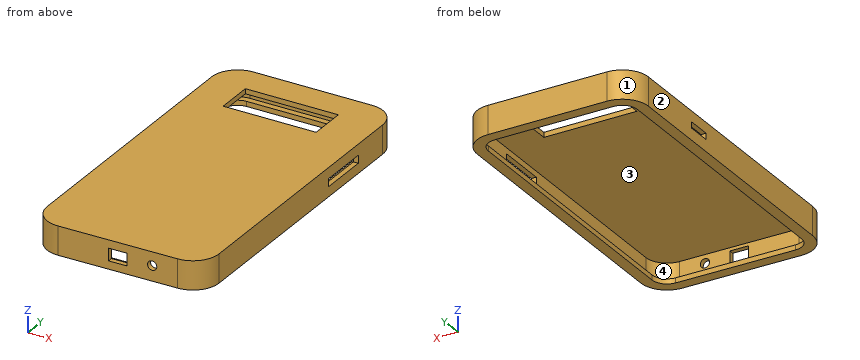
from build123d import *

# Parameters (mm, degrees)
F0_W       = 38.1
F0_H       = 15.24
F1_DEPTH   = 7.62
F2_W       = 20.32
F2_H       = 3.1982096843
F3_DEPTH   = 25.4
F5_W       = 10.16
F5_H       = 2.54
F6_DEPTH   = 25.4
F4_W       = 3.81
F4_H       = 5.08
F4_R       = 1.8758350377
F7_DEPTH   = 25.4
F8_DEPTH   = 7.62
F1_FACE3_W = 38.1
F1_FACE3_H = 15.24
F9_DEPTH   = 2.032
F10_DEPTH  = 2.032


with BuildPart() as f1:
    # F0 (on Top) → F1 (new body)
    with BuildSketch(Plane.XY):
        with BuildLine():
            Line((15.0151342493, 51.7147295177), (-33.7528657507, 51.7147295177))
            ThreePointArc((-33.7528657507, 51.7147295177), (-39.8594399131, 49.18530368), (-42.3888657507, 43.0787295177))
            Line((-42.3888657507, 43.0787295177), (-42.3888657507, -69.7396477934))
            ThreePointArc((-42.3888657507, -69.7396477934), (-39.8300752503, -75.8754460869), (-33.6700096372, -78.3752503123))
            Line((-33.6700096372, -78.3752503123), (15.0979903628, -77.9073354291))
            ThreePointArc((15.0979903628, -77.9073354291), (21.1509325427, -75.3489424097), (23.6511342493, -69.2717329101))
            Line((23.6511342493, -69.2717329101), (23.6511342493, 43.0787295177))
            ThreePointArc((23.6511342493, 43.0787295177), (21.1217084116, 49.18530368), (15.0151342493, 51.7147295177))
        make_face()
        with BuildLine():
            ThreePointArc((-39.8488657507, 43.0787295177), (-38.0633886888, 47.3892524558), (-33.7528657507, 49.1747295177))
            Line((-33.7528657507, 49.1747295177), (15.0151342493, 49.1747295177))
            ThreePointArc((15.0151342493, 49.1747295177), (19.3256571874, 47.3892524558), (21.1111342493, 43.0787295177))
            Line((21.1111342493, 43.0787295177), (21.1111342493, -69.2717329101))
            ThreePointArc((21.1111342493, -69.2717329101), (19.3462859858, -73.561527851), (15.0736209176, -75.3674523353))
            Line((15.0736209176, -75.3674523353), (-33.6943790824, -75.8353672185))
            ThreePointArc((-33.6943790824, -75.8353672185), (-38.0426606916, -74.07079953), (-39.8488657507, -69.7396477934))
            Line((-39.8488657507, -69.7396477934), (-39.8488657507, 43.0787295177))
        make_face(mode=Mode.SUBTRACT)
        with BuildLine():
            Line((15.0151342493, 49.1747295177), (-33.7528657507, 49.1747295177))
            ThreePointArc((-33.7528657507, 49.1747295177), (-38.0633886888, 47.3892524558), (-39.8488657507, 43.0787295177))
            Line((-39.8488657507, 43.0787295177), (-39.8488657507, -69.7396477934))
            ThreePointArc((-39.8488657507, -69.7396477934), (-38.0426606916, -74.07079953), (-33.6943790824, -75.8353672185))
            Line((-33.6943790824, -75.8353672185), (15.0736209176, -75.3674523353))
            ThreePointArc((15.0736209176, -75.3674523353), (19.3462859858, -73.561527851), (21.1111342493, -69.2717329101))
            Line((21.1111342493, -69.2717329101), (21.1111342493, 43.0787295177))
            ThreePointArc((21.1111342493, 43.0787295177), (19.3256571874, 47.3892524558), (15.0151342493, 49.1747295177))
        make_face()
        with Locations((-10.6388657507, 33.9347295177)):
            Rectangle(F0_W, F0_H, mode=Mode.SUBTRACT)
    extrude(amount=F1_DEPTH)

    # F2 (on face) → F3 (join)
    with BuildSketch(Plane.YZ.offset(23.6511342493)):
        with Locations((16.1547295177, 3.6192152184)):
            Rectangle(F2_W, F2_H)
    extrude(amount=F3_DEPTH)

    # F5 (on face) → F6 (join)
    with BuildSketch(Plane(origin=(-42.3888657507, 0, 0), x_dir=(0, -1, 0), z_dir=(-1, 0, 0))):
        with Locations((-8.5347295177, 4.0440695514)):
            Rectangle(F5_W, F5_H)
    extrude(amount=F6_DEPTH)

    # F4 (on face) → F7 (join)
    with BuildSketch(Plane(origin=(0.7488193587, -78.045011583, 0), x_dir=(0.9999539739, 0.0095942697, 0), z_dir=(0.0095942697, -0.9999539739, 0))):
        with Locations((-11.9402908808, 3.81)):
            Rectangle(F4_W, F4_H)
        with Locations((-8.1302908808, 3.81)):
            Rectangle(F4_W, F4_H)
        with Locations((3.9347091192, 4.1537573561)):
            Circle(F4_R)
    extrude(amount=F7_DEPTH)


with BuildPart() as f8:
    # F0 (on Top) → F8 (new body, through all)
    with BuildSketch(Plane.XY):
        with BuildLine():
            Line((15.0151342493, 53.7467295177), (-33.7528657507, 53.7467295177))
            ThreePointArc((-33.7528657507, 53.7467295177), (-41.2962808924, 50.6221446594), (-44.4208657507, 43.0787295177))
            Line((-44.4208657507, 43.0787295177), (-44.4208657507, -69.7396477934))
            ThreePointArc((-44.4208657507, -69.7396477934), (-41.2600068973, -77.3191633324), (-33.6505140811, -80.4071567873))
            Line((-33.6505140811, -80.4071567873), (15.1174859189, -79.9392419041))
            ThreePointArc((15.1174859189, -79.9392419041), (22.5946497883, -76.7788740567), (25.6831342493, -69.2717329101))
            Line((25.6831342493, -69.2717329101), (25.6831342493, 43.0787295177))
            ThreePointArc((25.6831342493, 43.0787295177), (22.558549391, 50.6221446594), (15.0151342493, 53.7467295177))
        make_face()
        with BuildLine():
            ThreePointArc((-42.3888657507, 43.0787295177), (-39.8594399131, 49.18530368), (-33.7528657507, 51.7147295177))
            Line((-33.7528657507, 51.7147295177), (15.0151342493, 51.7147295177))
            ThreePointArc((15.0151342493, 51.7147295177), (21.1217084116, 49.18530368), (23.6511342493, 43.0787295177))
            Line((23.6511342493, 43.0787295177), (23.6511342493, -69.2717329101))
            ThreePointArc((23.6511342493, -69.2717329101), (21.1509325427, -75.3489424097), (15.0979903628, -77.9073354291))
            Line((15.0979903628, -77.9073354291), (-33.6700096372, -78.3752503123))
            ThreePointArc((-33.6700096372, -78.3752503123), (-39.8300752503, -75.8754460869), (-42.3888657507, -69.7396477934))
            Line((-42.3888657507, -69.7396477934), (-42.3888657507, 43.0787295177))
        make_face(mode=Mode.SUBTRACT)
    extrude(amount=F8_DEPTH)

    # F8_face (on face) + F1_face3 (on face) → F9 (join)
    with BuildSketch(Plane(origin=(-9.4104092831, -13.214065849, 7.62), x_dir=(1, 0, 0), z_dir=(0, 0, 1))):
        with BuildLine():
            Line((35.0935435324, -56.0576670611), (35.0935435324, 56.2927953667))
            ThreePointArc((35.0935435324, 56.2927953667), (31.9689586741, 63.8362105084), (24.4255435324, 66.9607953667))
            Line((24.4255435324, 66.9607953667), (-24.3424564676, 66.9607953667))
            ThreePointArc((-24.3424564676, 66.9607953667), (-31.8858716093, 63.8362105084), (-35.0104564676, 56.2927953667))
            Line((-35.0104564676, 56.2927953667), (-35.0104564676, -56.5255819444))
            ThreePointArc((-35.0104564676, -56.5255819444), (-31.8495976142, -64.1050974834), (-24.240104798, -67.1930909383))
            Line((-24.240104798, -67.1930909383), (24.527895202, -66.7251760551))
            ThreePointArc((24.527895202, -66.7251760551), (32.0050590714, -63.5648082077), (35.0935435324, -56.0576670611))
        make_face()
        with BuildLine():
            ThreePointArc((-32.9784564676, 56.2927953667), (-30.4490306299, 62.399369529), (-24.3424564676, 64.9287953667))
            Line((-24.3424564676, 64.9287953667), (24.4255435324, 64.9287953667))
            ThreePointArc((24.4255435324, 64.9287953667), (30.5321176947, 62.399369529), (33.0615435324, 56.2927953667))
            Line((33.0615435324, 56.2927953667), (33.0615435324, -56.0576670611))
            ThreePointArc((33.0615435324, -56.0576670611), (30.5613418259, -62.1348765607), (24.5083996459, -64.69326958))
            Line((24.5083996459, -64.69326958), (-24.2596003541, -65.1611844633))
            ThreePointArc((-24.2596003541, -65.1611844633), (-30.4196659672, -62.6613802378), (-32.9784564676, -56.5255819444))
            Line((-32.9784564676, -56.5255819444), (-32.9784564676, 56.2927953667))
        make_face(mode=Mode.SUBTRACT)
    with BuildSketch(Plane(origin=(-9.3022040754, -16.6655356146, 7.62), x_dir=(1, 0, 0), z_dir=(0, 0, 1))):
        with BuildLine():
            ThreePointArc((32.9533383247, 59.7442651323), (30.423912487, 65.8508392946), (24.3173383247, 68.3802651323))
            Line((24.3173383247, 68.3802651323), (-24.4506616753, 68.3802651323))
            ThreePointArc((-24.4506616753, 68.3802651323), (-30.5572358376, 65.8508392946), (-33.0866616753, 59.7442651323))
            Line((-33.0866616753, 59.7442651323), (-33.0866616753, -53.0741121788))
            ThreePointArc((-33.0866616753, -53.0741121788), (-30.5278711749, -59.2099104723), (-24.3678055618, -61.7097146977))
            Line((-24.3678055618, -61.7097146977), (24.4001944382, -61.2417998145))
            ThreePointArc((24.4001944382, -61.2417998145), (30.4531366182, -58.6834067951), (32.9533383247, -52.6061972956))
            Line((32.9533383247, -52.6061972956), (32.9533383247, 59.7442651323))
        make_face()
        with Locations((-1.3366616753, 50.6002651323)):
            Rectangle(F1_FACE3_W, F1_FACE3_H, mode=Mode.SUBTRACT)
    extrude(amount=F9_DEPTH)

    # F0 (on Top) → F10 (join)
    with BuildSketch(Plane.XY):
        with BuildLine():
            Line((15.0151342493, 53.7467295177), (-33.7528657507, 53.7467295177))
            ThreePointArc((-33.7528657507, 53.7467295177), (-41.2962808924, 50.6221446594), (-44.4208657507, 43.0787295177))
            Line((-44.4208657507, 43.0787295177), (-44.4208657507, -69.7396477934))
            ThreePointArc((-44.4208657507, -69.7396477934), (-41.2600068973, -77.3191633324), (-33.6505140811, -80.4071567873))
            Line((-33.6505140811, -80.4071567873), (15.1174859189, -79.9392419041))
            ThreePointArc((15.1174859189, -79.9392419041), (22.5946497883, -76.7788740567), (25.6831342493, -69.2717329101))
            Line((25.6831342493, -69.2717329101), (25.6831342493, 43.0787295177))
            ThreePointArc((25.6831342493, 43.0787295177), (22.558549391, 50.6221446594), (15.0151342493, 53.7467295177))
        make_face()
        with BuildLine():
            ThreePointArc((-42.3888657507, 43.0787295177), (-39.8594399131, 49.18530368), (-33.7528657507, 51.7147295177))
            Line((-33.7528657507, 51.7147295177), (15.0151342493, 51.7147295177))
            ThreePointArc((15.0151342493, 51.7147295177), (21.1217084116, 49.18530368), (23.6511342493, 43.0787295177))
            Line((23.6511342493, 43.0787295177), (23.6511342493, -69.2717329101))
            ThreePointArc((23.6511342493, -69.2717329101), (21.1509325427, -75.3489424097), (15.0979903628, -77.9073354291))
            Line((15.0979903628, -77.9073354291), (-33.6700096372, -78.3752503123))
            ThreePointArc((-33.6700096372, -78.3752503123), (-39.8300752503, -75.8754460869), (-42.3888657507, -69.7396477934))
            Line((-42.3888657507, -69.7396477934), (-42.3888657507, 43.0787295177))
        make_face(mode=Mode.SUBTRACT)
        with BuildLine():
            Line((15.0151342493, 51.7147295177), (-33.7528657507, 51.7147295177))
            ThreePointArc((-33.7528657507, 51.7147295177), (-39.8594399131, 49.18530368), (-42.3888657507, 43.0787295177))
            Line((-42.3888657507, 43.0787295177), (-42.3888657507, -69.7396477934))
            ThreePointArc((-42.3888657507, -69.7396477934), (-39.8300752503, -75.8754460869), (-33.6700096372, -78.3752503123))
            Line((-33.6700096372, -78.3752503123), (15.0979903628, -77.9073354291))
            ThreePointArc((15.0979903628, -77.9073354291), (21.1509325427, -75.3489424097), (23.6511342493, -69.2717329101))
            Line((23.6511342493, -69.2717329101), (23.6511342493, 43.0787295177))
            ThreePointArc((23.6511342493, 43.0787295177), (21.1217084116, 49.18530368), (15.0151342493, 51.7147295177))
        make_face()
        with BuildLine():
            ThreePointArc((-39.8488657507, 43.0787295177), (-38.0633886888, 47.3892524558), (-33.7528657507, 49.1747295177))
            Line((-33.7528657507, 49.1747295177), (15.0151342493, 49.1747295177))
            ThreePointArc((15.0151342493, 49.1747295177), (19.3256571874, 47.3892524558), (21.1111342493, 43.0787295177))
            Line((21.1111342493, 43.0787295177), (21.1111342493, -69.2717329101))
            ThreePointArc((21.1111342493, -69.2717329101), (19.3462859858, -73.561527851), (15.0736209176, -75.3674523353))
            Line((15.0736209176, -75.3674523353), (-33.6943790824, -75.8353672185))
            ThreePointArc((-33.6943790824, -75.8353672185), (-38.0426606916, -74.07079953), (-39.8488657507, -69.7396477934))
            Line((-39.8488657507, -69.7396477934), (-39.8488657507, 43.0787295177))
        make_face(mode=Mode.SUBTRACT)
    extrude(amount=-F10_DEPTH)

    # F11: cut F1
    add(f1.part, mode=Mode.SUBTRACT)


solid = f8.part
CAD build for the part. Positions are in the model's coordinates, mm. Face numbers are marked on the shaded views. Give positions to 0.01 mm unless a question says otherwise; leave off trailing zeros. Loops run counter-clockwise (first coordinate to the right, second up) from the corner with the lowest first, then second, coordinate; pieces in that order, holes last. Notation, with made-up numbers: M -23.75,86.25 L 35.25,86.25 A4 cw 35.25,91.25 Z; hole C 13.5,-17.75 d11. An arc over 180 degrees is marked long. Answer in a Markdown table with one row per item. Add a question column.
Item 1: Mould opens along Y. For the marked faces 1, 2, 3 and 4 say: +Y half, -Y half, draft (parallel to the pull), parting line (faces both ways), or undercut.
Item 2: Band-saw the part on B-B on x = 1. Give the cut face in (y, z), then the cut area to 3 significant figures.
Item 3: Band-saw the part on C-C on y = 8.5. Give the cut face in (x, z), then the cut area to 3 significant figures.
Item 4: Band-saw the part on A-A on y = 33. Give the cut face in (x, z), then the cut area to 3 significant figures.
Item 5: Drop flat-ended pins along their axis: P1, Ø1, axis at x = -44, z = 4.5, coming from the +Y side; P2, Ø20, axis at x = -17.5, y = -33, coming from the -Z side; P3, Ø4, axis at x = 1, z = 2.5, coming from the -Y side. Give the stop position or say it passes through.
Item 6: Band-saw the part on D-D on x = -11.5. Give the cut face in (y, z).
Item 7: Probe probe 1 along X at (y, z) = (-65, 5.25); probe 2 along Y at (x, z) = (-12, 0.5); probe 3 along X at (y, z) = (-42.5, -0.25). List the from-to ranges inside material, lowest first.
Reply:
| question | item | result |
|---|---|---|
| 1 | face 1 | +Y half |
| 1 | face 2 | draft |
| 1 | face 3 | undercut |
| 1 | face 4 | undercut |
| 2 | outline | M -80.07,-2.03 L -75.5,-2.03 L -75.5,0 L -78.04,0 L -78.04,7.62 L 26.31,7.62 L 26.31,9.65 L -80.07,9.65 Z; M 41.55,7.62 L 51.71,7.62 L 51.71,0 L 49.17,0 L 49.17,-2.03 L 53.75,-2.03 L 53.75,9.65 L 41.55,9.65 Z |
| 2 | area | 291 mm^2 |
| 3 | outline | M -44.42,-2.03 L -39.85,-2.03 L -39.85,0 L -42.39,0 L -42.39,2.77 L -44.42,2.77 Z; M -44.42,5.31 L -42.39,5.31 L -42.39,7.62 L 23.65,7.62 L 23.65,5.22 L 25.68,5.22 L 25.68,9.65 L -44.42,9.65 Z; M 21.11,-2.03 L 25.68,-2.03 L 25.68,2.02 L 23.65,2.02 L 23.65,0 L 21.11,0 Z |
| 3 | area | 180 mm^2 |
| 4 | outline | M -44.42,-2.03 L -39.85,-2.03 L -39.85,0 L -42.39,0 L -42.39,7.62 L -29.69,7.62 L -29.69,9.65 L -44.42,9.65 Z; M 8.41,7.62 L 23.65,7.62 L 23.65,0 L 21.11,0 L 21.11,-2.03 L 25.68,-2.03 L 25.68,9.65 L 8.41,9.65 Z |
| 4 | area | 115 mm^2 |
| 5 | P1 | stops at y = 47.41 |
| 5 | P2 | stops at z = 7.62 |
| 5 | P3 | stops at y = -80.09 |
| 6 | outline | M -80.19,-2.03 L -75.62,-2.03 L -75.62,0 L -78.16,0 L -78.16,1.27 L -80.19,1.27 Z; M -80.19,6.35 L -78.16,6.35 L -78.16,7.62 L 26.31,7.62 L 26.31,9.65 L -80.19,9.65 Z; M 41.55,7.62 L 51.71,7.62 L 51.71,0 L 49.17,0 L 49.17,-2.03 L 53.75,-2.03 L 53.75,9.65 L 41.55,9.65 Z |
| 7 | probe 1 | x = -44.42 to -42.39, 23.65 to 25.68 |
| 7 | probe 2 | y = -80.2 to -78.17, 51.71 to 53.75 |
| 7 | probe 3 | x = -44.42 to -39.85, 21.11 to 25.68 |
